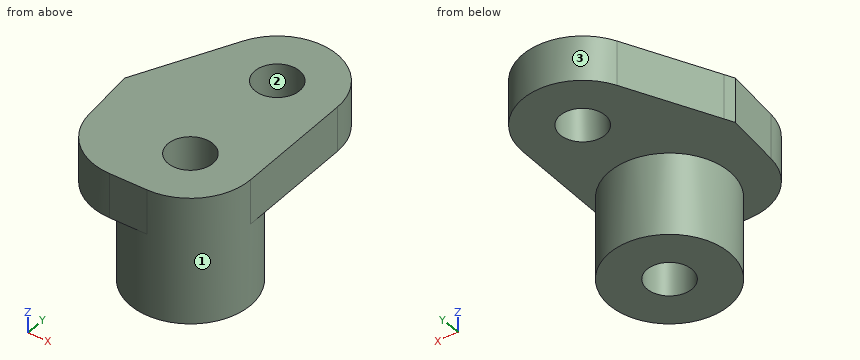
Autodesk Inventor part; units mm, degrees
ref_plane "YZ Plane" through (0, 0, 0) normal (1, 0, 0) x (0, 1, 0)
ref_plane "XZ Plane" through (0, 0, 0) normal (0, 1, 0) x (-1, 0, 0)
ref_plane "XY Plane" through (0, 0, 0) normal (0, 0, 1) x (1, 0, 0)
sketch "Skizze1" plane through (0, 0, 0) normal (0, 0, 1) x (1, 0, 0)
  circle A0 centre (0, 0) radius 4
  circle A1 centre (0, 8) radius 4
  line L0 (0, 0) -> (0, 8) construction
  line L1 (-4, 8) -> (-4, 0)
  line L2 (4, 0) -> (4, 8)
  dimension "d0" = 8
  dimension "d1" = 8
  dimension "d4" = 8
extrude "Extrusion1" add sketch "Skizze1" along normal blind 3
ref_plane "Arbeitsebene1" through (0, 8, 0) normal (1, 0, 0) x (0, 0, 1)
sketch "Skizze2" plane through (0, 0, 3) normal (0, 0, 1) x (1, 0, 0)
  arc A0 (-4, 0) -> (4, 0) centre (0, 0) ccw
  arc A1 (4, 8) -> (-4, 8) centre (0, 8) ccw
hole "Bohrung1" at (0, 8, 3) direction (0, 0, -1) diameter 3 end through all
hole "Bohrung2" at (0, 0, 3) direction (0, 0, -1) diameter 3 end through all
sketch "Skizze3" plane through (0, 0, 3) normal (0, 0, 1) x (1, 0, 0)
  arc A0 (-4, 0) -> (4, 0) centre (0, 0) ccw
  line L0 (4, 0) -> (4, 8)
  arc A1 (4, 8) -> (-4, 8) centre (0, 8) ccw
  line L1 (-6.5, 4) -> (-6.5, -4)
  line L2 (-6.5, -4) -> (0, -4)
  line L3 (-6.5, 4) -> (-3.570815, 9.802575)
  circle A2 centre (0, 0) radius 4 construction
  line L4 (0, 4) -> (-6.5, 4) construction
  circle A3 centre (0, 8) radius 1.5
  arc A4 (-4, 0) -> (4, 0) centre (0, 0) ccw
  circle A5 centre (0, 0) radius 1.5
  dimension "d16" = 6.5
extrude "Extrusion2" add sketch "Skizze3" against normal up to surface (3 mm away)
fillet "Rundung1" radius 4 1 edges at (-6.5, -4, 1.5)
sketch "Skizze4" plane through (0, 0, 0) normal (0, 0, -1) x (-1, 0, 0)
  arc A0 (-4, 0) -> (0, -4) centre (0, 0) ccw
  circle A1 centre (0, 0) radius 1.5
  circle A2 centre (0, 0) radius 4
  line L0 (6.5, 4) -> (0, 4)
  arc A3 (-4, 0) -> (0, -4) centre (0, 0) ccw
  circle A4 centre (0, 0) radius 1.5
  point P0 (3.18396, 8.32)
  point P1 (3.97995, 0.4)
sketch "Skizze4 outline for Extrusion3" plane through (0, 0, 0) normal (0, 0, -1) x (-1, 0, 0)
  circle A0 centre (0, 0) radius 4
  circle A1 centre (0, 0) radius 1.5
extrude "Extrusion3" add sketch "Skizze4 outline for Extrusion3" along normal blind 5.5
sketch "Skizze5" plane through (0, 0, 3) normal (0, 0, 1) x (1, 0, 0)
  arc A0 (-6.5, 0) -> (-2.5, -4) centre (-2.5, 0) ccw
  line L0 (-3.570815, 9.802575) -> (-6.5, 4)
  line L1 (-6.5, 4) -> (-6.5, 0)
  line L2 (-6.5, 4) -> (-6.811285, 3.383359)
  line L3 (-6.811285, 3.383359) -> (-6.484779, -0.348623)
  dimension "d26" = 5
extrude "Extrusion4" add sketch "Skizze5" against normal up to surface (3 mm away)
equation "\"d0\" = Finger_diameter"
equation "\"d1\" = d0"
equation "\"d4\" = d0"
equation "\"d2\" = Join_width"
equation "\"d5\" = bearingHole"
equation "\"d19\" = bearingHole"
equation "\"FingerLaenge_B\" = 25"
equation "\"Hebel_B\" = 25"
equation "\"Finger_width\" = 22"
equation "\"Finger_diameter\" = 8"
equation "\"FingerWall\" = 3"
equation "\"Hebel_basis_2\" = 15"
equation "\"Join_width\" = 3"
equation "\"bearingHole\" = 3"
equation "\"bearingWall\" = 4"
equation "\"support_D\" = 0.25"
properties part number "FingerTip_joint _v2"
Could you check a few things on this model? Use its own coordinates, in mm. Face numbers are marked on the shaded views. Round coordinates to 2 decimals unless told otherwise and drop trailing zeros. Loops run counter-clockwise (first coordinate to the right, second up) from the corner with the lowest first, then second, coordinate; pieces in that order, holes last. Notation, with made-up numbers: (67, -21) -> (123, -21) arc R23 cw to (123, -12) -> close; hole circle Ø6 at (58.5, 67.5). An arc over 180 degrees is marked (long way). Put each result on its own line as item: value.
Q1. I want a section at A-A on z = 0.25. Write out the boundary of the cut face in (x, y), and give its area (3 significant figures).
Checks:
outline: (-6.81, 3.38) -> (-6.48, -0.35) arc R4 ccw to (-2.5, -4) -> (0, -4) arc R4 ccw to (4, 0) -> (4, 8) arc R4 ccw to (-3.57, 9.8) -> (-6.5, 4) -> close; hole circle Ø3 at (0, 0); hole circle Ø3 at (0, 8)
area: 127 mm2
Q2. For pin 1 Ø2 at (y, z) = (4.5, -0.5) entering from -X; pin 2 Ø5.5 at (x, y) = (0.5, 7.5) entering from -Z; pin 3 Ø2 at (x, z) = (1.5, -4) entering from +Y, each with a flat end and sliding along its axis, tell me the tip position at first contact or that it passes through.
Checks:
pin 1: x = -6.68
pin 2: z = 0
pin 3: y = 3.97
Q3. Please list where these lines run through material, in increasing order: line 1 (Y direction, x = 0, z = 1); line 2 (Y direction, x = 0, z = -2.5). Write a range as from..to.
Checks:
line 1: -4..-1.5, 1.5..6.5, 9.5..12
line 2: -4..-1.5, 1.5..4
Q4. I want a section at B-B on x = 0.5. Write out the boundary of the cut face in (y, z).
Checks:
outline: (-3.97, -5.5) -> (-1.41, -5.5) -> (-1.41, 3) -> (-3.97, 3) -> close; (1.41, -5.5) -> (3.97, -5.5) -> (3.97, 0) -> (6.59, 0) -> (6.59, 3) -> (1.41, 3) -> close; (9.41, 0) -> (11.97, 0) -> (11.97, 3) -> (9.41, 3) -> close
Q5. Thinking about a two-plate mould opening in Y: for the marked faces 1, 2 and 3, which applies, pulls with the +Y half, pulls with the -Y half, needs draft (parallel to the pull), parting line crosses it, or undercut?
Checks:
face 1: parting line crosses it
face 2: undercut
face 3: pulls with the +Y half
Q6. I want a section at D-D on x = -1. Write out the boundary of the cut face in (y, z).
Checks:
outline: (-4, 0) -> (-3.87, 0) -> (-3.87, -5.5) -> (-1.12, -5.5) -> (-1.12, 3) -> (-4, 3) -> close; (1.12, -5.5) -> (3.87, -5.5) -> (3.87, 0) -> (6.88, 0) -> (6.88, 3) -> (1.12, 3) -> close; (9.12, 0) -> (11.87, 0) -> (11.87, 3) -> (9.12, 3) -> close
Q7. I want a section at C-C on z = -0.75. Write out the boundary of the cut face in (x, y).
Checks:
outline: circle Ø8 at (0, 0); hole circle Ø3 at (0, 0)
